Geometry: final body of the model. Coordinates: model frame, mm. Round coordinates to 2 decimals unless told otherwise and drop trailing zeros. Write each loop counter-clockwise with the first axis right and the second up, starting at its lowest first coordinate (ties: lowest second). Pieces come first, ordered by that corner, then holes. Notation, with made-up numbers: M 24.5,2 L 37.5,2 A18 cw 37.5,26 Z; hole C -11.75,63 d11. An arc over 180 degrees is marked long. Put each result on its own line as item: value. Start each with the question number.
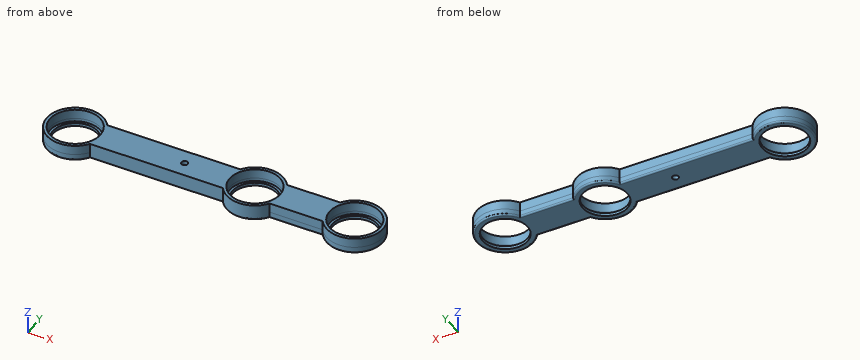
```python
from build123d import *

# Parameters (mm, degrees)
BOSS_EXTRU_1_DEPTH      = 4
ESQUISSE6_R             = 16
ENL_V_MAT_EXTRU_1_DEPTH = 2
ESQUISSE7_R             = 14.25
ENL_V_MAT_EXTRU_2_DEPTH = 135.227418958
ESQUISSE10_R            = 16
BOSS_EXTRU_5_DEPTH      = 6
CONG_1_R                = 1
ESQUISSE12_R            = 2
ENL_V_MAT_EXTRU_3_DEPTH = 135.58454603


with BuildPart() as part:
    # Esquisse1 → Boss.-Extru.1 (new body)
    with BuildSketch(Plane.XY):
        with BuildLine():
            Line((-100.033370453, 10), (-14.966629547, 10))
            ThreePointArc((-14.966629547, 10), (0, 18), (14.966629547, 10))
            Line((14.966629547, 10), (48.933370453, 10))
            ThreePointArc((48.933370453, 10), (81.9, 0), (48.933370453, -10))
            Line((48.933370453, -10), (14.966629547, -10))
            ThreePointArc((14.966629547, -10), (0, -18), (-14.966629547, -10))
            Line((-14.966629547, -10), (-100.033370453, -10))
            ThreePointArc((-100.033370453, -10), (-133, 0), (-100.033370453, 10))
        make_face()
    extrude(amount=BOSS_EXTRU_1_DEPTH)

    # Esquisse6 → Enlèv. mat.-Extru.1 (cut)
    with BuildSketch(Plane.XY.offset(4)):
        with Locations((-115, 0)):
            Circle(ESQUISSE6_R)
        Circle(ESQUISSE6_R)
        with Locations((63.9, 0)):
            Circle(ESQUISSE6_R)
    extrude(amount=-ENL_V_MAT_EXTRU_1_DEPTH, mode=Mode.SUBTRACT)

    # Esquisse7 → Enlèv. mat.-Extru.2 (cut, through all)
    with BuildSketch(Plane.XY.offset(2)):
        with Locations((-115, 0)):
            Circle(ESQUISSE7_R)
        Circle(ESQUISSE7_R)
        with Locations((63.9, 0)):
            Circle(ESQUISSE7_R)
    extrude(amount=-ENL_V_MAT_EXTRU_2_DEPTH, mode=Mode.SUBTRACT)

    # Esquisse10 → Boss.-Extru.5 (add)
    with BuildSketch(Plane.XY.offset(4)):
        with BuildLine():
            Line((-100.033370453, -10), (-14.966629547, -10))
            ThreePointArc((-14.966629547, -10), (0, -18), (14.966629547, -10))
            Line((14.966629547, -10), (48.933370453, -10))
            ThreePointArc((48.933370453, -10), (81.9, 0), (48.933370453, 10))
            Line((48.933370453, 10), (14.966629547, 10))
            ThreePointArc((14.966629547, 10), (0, 18), (-14.966629547, 10))
            Line((-14.966629547, 10), (-100.033370453, 10))
            ThreePointArc((-100.033370453, 10), (-133, 0), (-100.033370453, -10))
        make_face()
        with Locations((63.9, 0)):
            Circle(ESQUISSE10_R, mode=Mode.SUBTRACT)
        Circle(ESQUISSE10_R, mode=Mode.SUBTRACT)
        with Locations((-115, 0)):
            Circle(ESQUISSE10_R, mode=Mode.SUBTRACT)
    extrude(amount=BOSS_EXTRU_5_DEPTH)

    # Congé1
    cong_1_edges = [part.edges().sort_by_distance(p)[0] for p in [
        (31.95, -10, 0),
        (0, -18, 0),
        (-57.5, -10, 0),
        (-133, 0, 0),
        (-57.5, 10, 0),
        (0, 18, 0),
        (31.95, 10, 0),
        (81.9, 0, 0),
    ]]
    fillet(cong_1_edges, radius=CONG_1_R)

    # Esquisse12 → Enlèv. mat.-Extru.3 (cut, through all)
    with BuildSketch(Plane(origin=(0, 0, 0), x_dir=(-1, 0, 0), z_dir=(0, 0, -1))):
        with Locations((45, 0)):
            Circle(ESQUISSE12_R)
    extrude(amount=-ENL_V_MAT_EXTRU_3_DEPTH, mode=Mode.SUBTRACT)


solid = part.part
```
1) Ray query, probe 1 along X at (y, z) = (13.5, 8); probe 2 along Y at (x, z) = (-45, 4.5); probe 3 along X at (y, z) = (-3, 6.5). Return the intervals inside material, ascending.
2) Section C-C, the plane z = 7.5. Output: boundary loops of the cut face in (x, y), and give its area (3 significant figures).
3) First-contact query: pin 1 (5 mm diameter, centred on x = 31, z = 8.5, fed in from -Y); pin 2 (4 mm diameter, centred on x = 1, y = -11.5, fed in from +Z); pin 3 (4 mm diameter, centred on y = -9.5, z = 8.5, fed in from -X); pin 4 (5 mm diameter, centred on x = -61.5, z = 8, fed in from +Y). Flat tips, straight axial feed; report the tip coordinate or a pass-through.
4) Section D-D, the plane x = -45. Output: boundary loops of the cut face in (y, z).
5) Section B-B, the plane y = 0. Give the number of separate pieces and of enclosed holes in the cut face, and give its area (3 significant figures).
6) Section A-A, the plane x = 0. Output: boundary loops of the cut face in (y, z).
Solved:
1. probe 1: x = -126.91 to -123.59, -106.41 to -103.09, -11.91 to -8.59, 8.59 to 11.91, 51.99 to 55.31, 72.49 to 75.81
1. probe 2: y = -10 to -2, 2 to 10
1. probe 3: x = -132.75 to -130.72, -99.28 to -15.72, 15.72 to 48.18, 79.62 to 81.65
2. outline: M -100.03,-10 L -14.97,-10 A18 ccw 14.97,-10 L 48.93,-10 A18 ccw long 48.93,10 L 14.97,10 A18 ccw -14.97,10 L -100.03,10 A18 ccw long Z; hole C -115,0 d32; hole C -45,0 d4; hole C 0,0 d32; hole C 63.9,0 d32
2. area: 2,840 mm2
3. pin 1: stops at y = -10
3. pin 2: passes through
3. pin 3: stops at x = -131.36
3. pin 4: stops at y = 10
4. outline: M -10,1 A1 ccw -9,0 L -2,0 L -2,10 L -10,10 Z; M 2,0 L 9,0 A1 ccw 10,1 L 10,10 L 2,10 Z
5. separate pieces: 5
5. enclosed holes: 0
5. area: 1,170 mm2
6. outline: M -18,1 A1 ccw -17,0 L -14.25,0 L -14.25,2 L -16,2 L -16,10 L -18,10 Z; M 14.25,0 L 17,0 A1 ccw 18,1 L 18,10 L 16,10 L 16,2 L 14.25,2 Z
